Study the drawing (mm; zero at the part's minimum x, y, z) and answer. Give positions to 0.01 mm unless a question says otherwise; leave off trailing zeros. Order: outer loops, then holes, each group sorted by start corner. A loop starts at its lowest first (then second) coordinate and runs counter-clockwise, first axis right, second up.
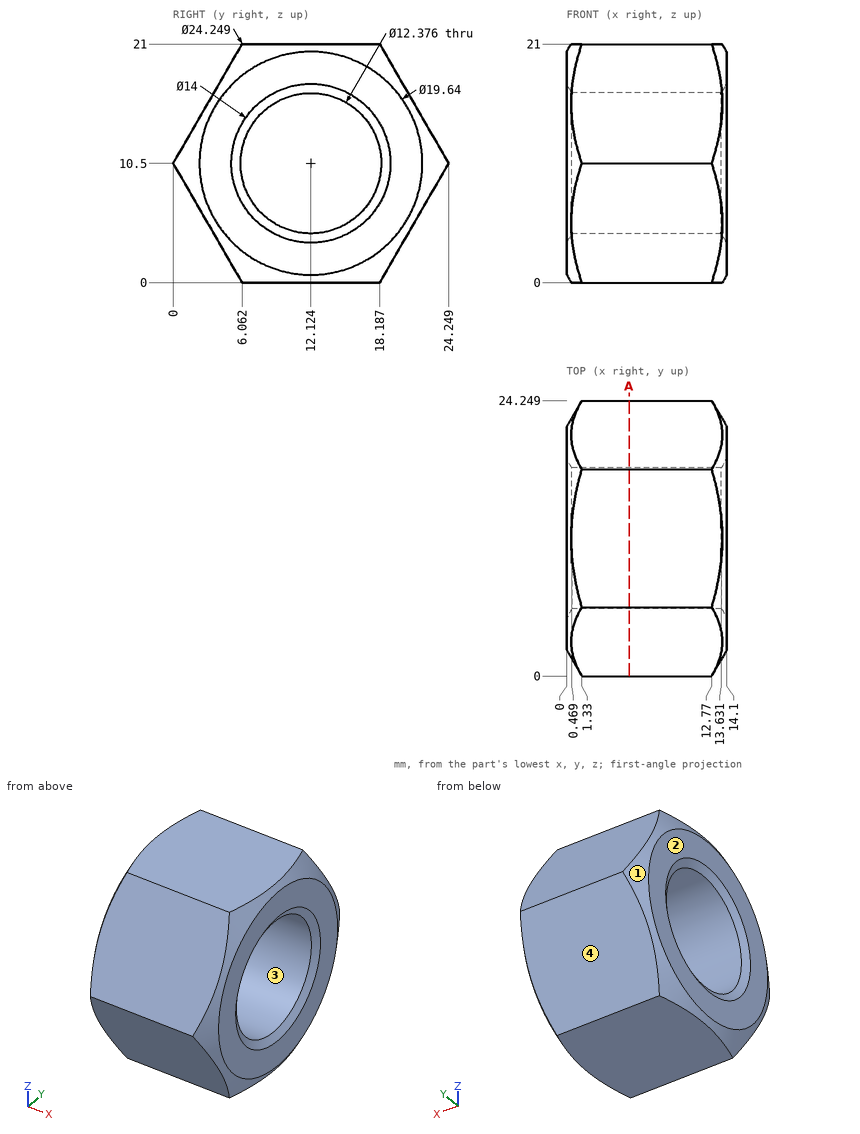
1) Given P1, Ø2, axis at x = 3, z = 7, coming from the -Y side; P2, Ø4, axis at x = 9.5, z = 15, coming from the +Y side (1 decimal); P3, Ø5, axis at x = 10, z = 14, coming from the -Y side, each flat-ended and moving along its own axis, determine where each tip first touches the part or whether it passes through.
Geometry says:
P1: stops at y = 1.44
P2: stops at y = 22.8
P3: stops at y = 0.58
2) Find section A-A (x = 5.5). Write down the section's boundary in (y, z) (1 decimal).
Geometry says:
outline: (0, 10.5) - (6.1, 0) - (18.2, 0) - (24.2, 10.5) - (18.2, 21) - (6.1, 21) - close; hole circle Ø12.4 at (12.1, 10.5)
3) Straight lines are drawn through the part: probe 1 along Z at (x, y) = (3.75, 11.5); probe 2 along Z at (x, y) = (4.5, 10.5); probe 3 along Y at (x, z) = (11.5, 11) (1 decimal). For each, find the intervals that lie inside material, in ascending order.
Geometry says:
probe 1: z = 0 to 4.34, 16.66 to 21
probe 2: z = 0 to 4.53, 16.47 to 21
probe 3: y = 0.3 to 6, 18.3 to 24
4) For a pull along Y with two mould halves and no side action, classify the marked faces 1, 2, 3 and 4 as +Y half, -Y half, draft (parallel to the pull), parting line (faces both ways), or undercut.
Geometry says:
face 1: parting line
face 2: draft
face 3: undercut
face 4: +Y half
